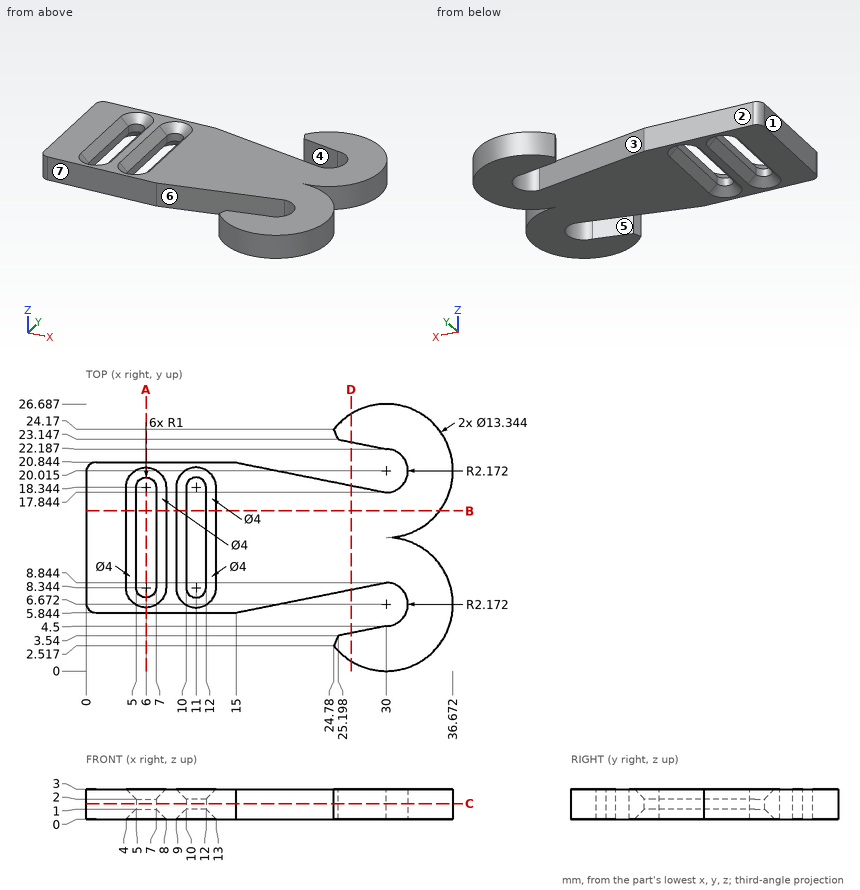
For this review, use the dimensioned drawing (mm, ordinates from the lowest corner) and the shaded views. A direction names the side the tool comes from. Round coordinates to 2 decimals unless told otherwise and drop trailing zeros. Order: outer loops, then holes, each group sorted by start corner. A loop starts at its lowest first (then second) coordinate and runs counter-clockwise, first axis right, second up. Notation, with made-up numbers: (-36.5, -23.75) -> (-20.5, -23.75) arc R18 ccw to (-20.5, 6.25) -> close; hole circle Ø7 at (30.25, 78.5). An arc over 180 degrees is marked (long way). Put each result on its own line as item: value.
Q1. Insertion check: pin 1 Ø0.9 at (x, z) = (10.5, 2) entering from +Y; pin 2 Ø1.1 at (y, z) = (12, 1.5) entering from +X (1 decimal). Each pin has a flat end and moves straight along its axis. Give the tip position at first contact, or say it passes through.
Check result:
pin 1: y = 20.84
pin 2: x = 34.7
Q2. Machinability: for the marked faces 1, 2, 3 and 4, which of the approach directions +Z, -Z, +X, -X, +Y, -Y give a long, thin tool a straight path to every point of the face, cutting with its end or side? Answer none if there is none.
Check result:
face 1: +Z, -Z, -X, +Y, -Y
face 2: +Z, -Z, -X, +Y
face 3: +Z, -Z
face 4: +Z, -Z, -X
Q3. For probe 1 along X at (y, z) = (12, 0.6) (1 decimal); probe 2 along X at (y, z) = (15, 1.5); probe 3 along Y at (x, z) = (11, 1.05), list the stretches that pass through material, from the lowest coordinate up. Write a range as [from, to].
Check result:
probe 1: [0, 4.6], [7.4, 9.6], [12.4, 34]
probe 2: [0, 5], [7, 10], [12, 34.4]
probe 3: [5.84, 7.34], [19.34, 20.84]
Q4. Add section A-A on x = 6. Write out the cut boundary in (y, z).
Check result:
outline: (5.84, 0) -> (6.34, 0) -> (7.34, 1) -> (7.34, 2) -> (6.34, 3) -> (5.84, 3) -> close; (19.34, 1) -> (20.34, 0) -> (20.84, 0) -> (20.84, 3) -> (20.34, 3) -> (19.34, 2) -> close
Q5. Add section D-D on x = 26.5. Write out the cut boundary in (y, z) (1 decimal).
Check result:
outline: (1, 0) -> (3.8, 0) -> (3.8, 3) -> (1, 3) -> close; (8.1, 0) -> (18.5, 0) -> (18.5, 3) -> (8.1, 3) -> close; (22.9, 0) -> (25.7, 0) -> (25.7, 3) -> (22.9, 3) -> close
Q6. Mouldability with a two-part tool opening along X and no side actions: class the marked faces 5, 6 and 7 as pulls with the +X half, pulls with the -X half, needs draft (parallel to the pull), parting line crosses it, or undercut.
Check result:
face 5: pulls with the -X half
face 6: undercut
face 7: needs draft
Q7. Add section B-B on y = 16. Write out the cut boundary in (x, z).
Check result:
outline: (0, 0) -> (4, 0) -> (5, 1) -> (5, 2) -> (4, 3) -> (0, 3) -> close; (7, 1) -> (8, 0) -> (9, 0) -> (10, 1) -> (10, 2) -> (9, 3) -> (8, 3) -> (7, 2) -> close; (12, 1) -> (13, 0) -> (35.33, 0) -> (35.33, 3) -> (13, 3) -> (12, 2) -> close
Q8. Add section C-C on z = 1.55. Write out the cut boundary in (x, y) (1 decimal).
Check result:
outline: (0, 6.8) arc R1 ccw to (1, 5.8) -> (15, 5.8) -> (30, 8.8) arc R2.2 cw to (30, 4.5) -> (25.2, 3.5) -> (24.8, 2.5) arc R6.7 ccw (long way) to (30, 13.3) arc R6.7 ccw (long way) to (24.8, 24.2) -> (25.2, 23.1) -> (30, 22.2) arc R2.2 cw to (30, 17.8) -> (15, 20.8) -> (1, 20.8) arc R1 ccw to (0, 19.8) -> close; hole (5, 8.3) arc R1 ccw to (7, 8.3) -> (7, 18.3) arc R1 ccw to (5, 18.3) -> close; hole (10, 8.3) arc R1 ccw to (12, 8.3) -> (12, 18.3) arc R1 ccw to (10, 18.3) -> close
